Verification items for this drawing (mm, ordinates from the low corner). A direction names the side the tool comes from. Round coordinates to 2 decimals unless told otherwise and drop trailing zeros. Order: outer loops, then holes, each group sorted by start corner. A loop starts at its lowest first (then second) coordinate and runs counter-clockwise, first axis right, second up. Notation, with made-up numbers: M -12.5,-24 L 13.5,-24 A7 cw 13.5,-14 Z; hole C -37,48 d5. An arc over 180 degrees is marked long. Use CSV: the item, a comma, the result in double quotes. Start each with the question number.
Q1. Set-up check for the marked faces 1 and 2: record each of +Z, -Z, +X, -X, +Y, -Y from which the full face is reachable in a straight line by a thin tool's end or side.
Q2. Gauge pin test, flat ends, axial feed: pin 1 Ø6 at (x, z) = (70.5, 16) entering from +Y; pin 2 Ø12 at (x, z) = (77.5, 18.5) entering from -Y; pin 3 Ø1.5 at (y, z) = (1.5, 19) entering from +X; pin 4 Ø0.9 at (x, y) = (216, 1.5) entering from +Z. Record the tip position at first contact, or that the pin passes through.
Q3. Sectioned sample at A-A (z = 7.25). Enter the section's corners in (x, y), and give its area (3 significant figures).
Q4. Scan line: line 1 (Y direction, x = 163, z = 11.5). Record every from-to range of solid material in increasing order.
Q5. Sectioned sample at B-B (x = 33). Enter the section's corners in (y, z), and give its area (3 significant figures).
Q6. Sectioned sample at D-D (x = 96.5). Enter the section's corners in (y, z), and give its area (3 significant figures).
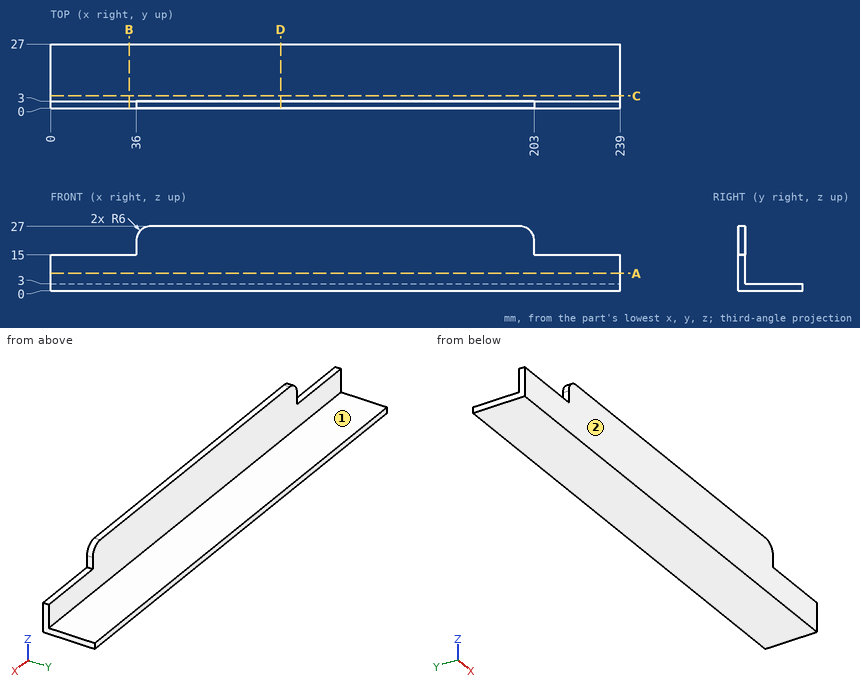
Verdict:
1,face 1,"+Z, +X, -X, +Y"
1,face 2,"+Z, -Z, +X, -X, -Y"
2,pin 1,"stops at y = 3"
2,pin 2,"stops at y = 0"
2,pin 3,"stops at x = 203"
2,pin 4,"stops at z = 15"
3,outline,"M 0,0 L 239,0 L 239,3 L 0,3 Z"
3,area,"717 mm²"
4,line 1,"y = 0 to 3"
5,outline,"M 0,0 L 27,0 L 27,3 L 3,3 L 3,15 L 0,15 Z"
5,area,"117 mm²"
6,outline,"M 0,0 L 27,0 L 27,3 L 3,3 L 3,27 L 0,27 Z"
6,area,"153 mm²"
